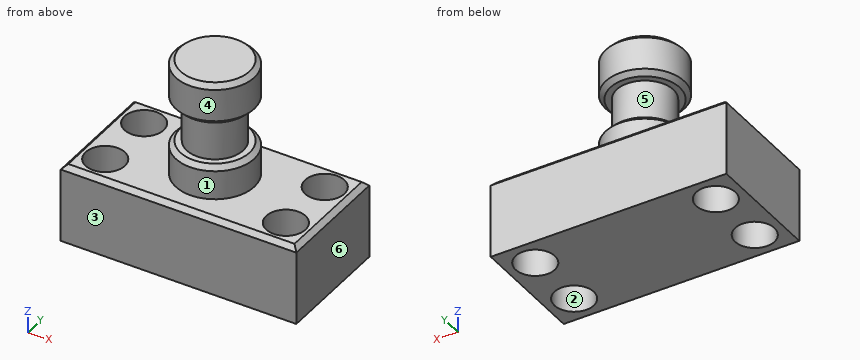
```python
from build123d import *

# Parameters (mm, degrees)
F0_W     = 76.2
F0_H     = 38.1
F1_DEPTH = 25.4
F2_R     = 6.35
F3_DEPTH = 25.4
F4_DEPTH = 25.4
F5_R     = 12.7
F6_DEPTH = 38.1
F7_W     = 16.6140981019
F7_H     = 13.6993415654
F9_SIZE  = 1.524
F10_SIZE = 1.524
F11_SIZE = 1.524


with BuildPart() as f1:
    # F0 (on Top) → F1 (new body)
    with BuildSketch(Plane.XY):
        with Locations((2.8314734757, -25.9829519808)):
            Rectangle(F0_W, F0_H)
    extrude(amount=F1_DEPTH)

    # F2 (on Top) → F3 (cut)
    with BuildSketch(Plane.XY):
        with Locations((-26.3785265243, -15.8229519808)):
            Circle(F2_R)
    extrude(amount=F3_DEPTH, mode=Mode.SUBTRACT)

    # F2 (on Top) → F4 (cut)
    with BuildSketch(Plane.XY):
        with Locations((-26.3785265243, -15.8229519808)):
            Circle(F2_R)
        with Locations((-26.3785265243, -36.1429519808)):
            Circle(F2_R)
        with Locations((32.0414734757, -15.8229519808)):
            Circle(F2_R)
        with Locations((32.0414734757, -36.1429519808)):
            Circle(F2_R)
    extrude(amount=F4_DEPTH, mode=Mode.SUBTRACT)

    # F5 (on face) → F6 (join)
    with BuildSketch(Plane.XY.offset(25.4)):
        with Locations((2.8314734757, -25.9829519808)):
            Circle(F5_R)
    extrude(amount=F6_DEPTH)

    # F7 (on Right) → F8 (revolve, cut)
    with BuildSketch(Plane.YZ):
        with Locations((-42.9926235229, 43.1383606046)):
            Rectangle(F7_W, F7_H)
    revolve(axis=Axis((2.8314734757, -25.9829519808, 63.5), (0, 0, 1)), mode=Mode.SUBTRACT)

    # F9
    f9_edges = [f1.edges().sort_by_distance(p)[0] for p in [
        (40.931473, -25.982952, 25.4),
    ]]
    chamfer(f9_edges, length=F9_SIZE)

    # F10
    f10_edges = [f1.edges().sort_by_distance(p)[0] for p in [
        (2.069473, -6.932952, 25.4),
        (-35.268527, -25.982952, 25.4),
    ]]
    chamfer(f10_edges, length=F10_SIZE)

    # F11
    f11_edges = [f1.edges().sort_by_distance(p)[0] for p in [
        (2.831473, -45.032952, 25.4),
        (-9.868527, -25.982952, 36.28869),
        (-9.868527, -25.982952, 49.988031),
        (-9.868527, -25.982952, 63.5),
    ]]
    chamfer(f11_edges, length=F11_SIZE)


solid = f1.part
```
Input: part model. Units: mm. Frame: model coordinates. Face numbers are marked on the shaded views. A direction names the side the tool comes from. Give positions to 0.01 mm unless a question says otherwise; leave off trailing zeros. Order: outer loops, then holes, each group sorted by start corner. A loop starts at its lowest first (then second) coordinate and runs counter-clockwise, first axis right, second up. Notation, with made-up numbers: (65.5, 43) - (82.5, 43) arc R12 cw to (82.5, 64) - close; hole circle Ø2 at (74, 58). An arc over 180 degrees is marked (long way). Use a Markdown table: item, result.
(1) Pin query (flat end, axial travel): pin 1 (8 mm diameter, centred on y = -21.5, z = 37.5, fed in from -X); pin 2 (11.5 mm diameter, centred on x = 32.04, y = -15.82, fed in from -Z); pin 3 (20.5 mm diameter, centred on x = -26.38, y = -36.14, fed in from +Z); pin 4 (10 mm diameter, centred on y = -26.5, z = 47.5, fed in from +X). Return the tip coordinate at first contact, or that it passes through.
Computed values:
| item | result |
|---|---|
| pin 1 | stops at x = -9.77 |
| pin 2 | passes through |
| pin 3 | stops at z = 25.4 |
| pin 4 | stops at x = 15.53 |
(2) Section query A-A (y = -40.5). Output: boundary loops of the cut face in (x, z).
Computed values:
| item | result |
|---|---|
| outline | (-35.27, 0) - (-31, 0) - (-31, 25.4) - (-33.74, 25.4) - (-35.27, 23.88) - close; (-21.76, 0) - (27.42, 0) - (27.42, 25.4) - (-21.76, 25.4) - close; (36.66, 0) - (40.93, 0) - (40.93, 23.88) - (39.41, 25.4) - (36.66, 25.4) - close |
(3) Section query B-B (x = 29). Output: boundary loops of the cut face in (y, z).
Computed values:
| item | result |
|---|---|
| outline | (-45.03, 0) - (-41.72, 0) - (-41.72, 25.4) - (-43.51, 25.4) - (-45.03, 23.88) - close; (-30.57, 0) - (-21.4, 0) - (-21.4, 25.4) - (-30.57, 25.4) - close; (-10.25, 0) - (-6.93, 0) - (-6.93, 23.88) - (-8.46, 25.4) - (-10.25, 25.4) - close |
(4) Section query C-C (z = 11.5). Output: boundary loops of the cut face in (x, y).
Computed values:
| item | result |
|---|---|
| outline | (-35.27, -45.03) - (40.93, -45.03) - (40.93, -6.93) - (-35.27, -6.93) - close; hole circle Ø12.7 at (-26.38, -36.14); hole circle Ø12.7 at (-26.38, -15.82); hole circle Ø12.7 at (32.04, -36.14); hole circle Ø12.7 at (32.04, -15.82) |
(5) Draft query along Y for the marked faces 1, 2 and 3. Return one class per face: released by +Y, released by -Y, zero draft, split by the parting line, or undercut.
Computed values:
| item | result |
|---|---|
| face 1 | split by the parting line |
| face 2 | undercut |
| face 3 | released by -Y |
(6) Access query for the marked faces 4, 5 and 6. Directions: +Z, -Z, +X, -X, +Y, -Y. A direction counts if a zero-diameter tool reaches every point of the face in a straight line with its end or side. Return the directions, or none.
Computed values:
| item | result |
|---|---|
| face 4 | +Z |
| face 5 | none |
| face 6 | +Z, -Z, +X, +Y, -Y |
(7) Section query D-D (z = 41). Output: boundary loops of the cut face in (x, y).
Computed values:
| item | result |
|---|---|
| outline | circle Ø18.3 at (2.83, -25.98) |
(8) Line query: line 1 (X direction, y = -36.5, z = 9.5); line 2 (Y direction, x = 35, z = 16.5); line 3 (X direction, y = -31, z = 13). Output: solid intervals per line, ascending. Write a range as from..to.
Computed values:
| item | result |
|---|---|
| line 1 | x = -35.27..-32.72, -20.04..25.7, 38.38..40.93 |
| line 2 | y = -45.03..-41.76, -30.52..-21.44, -10.2..-6.93 |
| line 3 | x = -35.27..-30.1, -22.65..28.32, 35.77..40.93 |
